Read the model definition and answer for the solid it produces. Units are mm, in the model's axes. A direction names the side the tool comes from. Coordinates: 2 decimals unless noted, no trailing zeros. Write each loop counter-clockwise with the first axis right and the second up, starting at its lowest first coordinate (ties: lowest second). Pieces come first, ordered by that corner, then holes.
from build123d import *

# Parameters (mm, degrees)
F1_DEPTH = 25.4


with BuildPart() as f1:
    # F0 (on Top) → F1 (new body)
    with BuildSketch(Plane.XY):
        Polygon((99.490069, 58.291368), (98.893963, 58.039229), (98.893963, 12.895242), (100.236297, 13.898268), (98.893963, 12.464104), (98.893963, -29.808243), (102.997907, -27.43528), (98.893963, -31.945548), (98.893963, -111.925168), (99.639752, -112.016652), (120.770343, 120.569244), (-22.619633, 111.361951), (105.815612, 95.447481), align=None)
        Polygon((98.893963, 12.895242), (98.893963, 58.039229), (-38.321942, 0), (97.543553, 35.373725), (5.177082, -57.132415), align=None)
        Polygon((100.236297, 13.898268), (98.893963, 12.895242), (98.893963, 12.464104), align=None)
        Polygon((98.893963, -29.808243), (98.893963, 12.464104), (12.658387, -79.670966), align=None)
        Polygon((102.997907, -27.43528), (98.893963, -29.808243), (98.893963, -31.945548), align=None)
        Polygon((98.893963, -111.925168), (98.893963, -31.945548), (33.426806, -103.894494), align=None)
        Polygon((99.639752, -112.016652), (98.893963, -111.925168), (98.893963, -120.225601), align=None)
    extrude(amount=F1_DEPTH)


solid = f1.part
Item 1: Find the intervals of material crossed by probe 1 along Y at (x, z) = (88, 15) (3 decimals); probe 2 along Y at (x, z) = (8.5, 14.25); probe 3 along Y at (x, z) = (92, 2), in increasing order.
Item 2: The part is cut by section B-B (y = -27). Give the vertices of the cut face in (x, z).
Item 3: Determine the mould class of faces 1 (the flat face through (82, 1, 25.4)), 2 (the flat face through (65.702, -107.854, 12.522)), 3 (the flat face through (52.01, -10.23, 12.52)) for opening direction Y: +Y half, -Y half, draft (parallel to the pull), parting line (faces both ways), or undercut.
Item 4: Given pin 1 (1.7 mm diameter, centred on y = -30.5, z = 8.5, fed in from -X); pin 2 (0.5 mm diameter, centred on y = 12.5, z = 17.5, fed in from -X); pin 3 (6 mm diameter, centred on x = 61, z = 20.5, fed in from +Y); pin 4 (6 mm diameter, centred on x = 68.5, y = -24, fed in from -Z), each flat-ended and moving along its own axis, determine where each tip first touches the part or whether it passes through.
Item 5: The part is cut by section A-A (x = -4). Give the vertices of the cut face in (y, z), and give its area (3 significant figures).
Item 6: The part is cut by section D-D (x = 82.5). Give the vertices of the cut face in (y, z), and give its area (3 significant figures).
Item 7: For faces 4 (the flat face through (82, 1, 0)), 5 (the flat face through (51.38, -22.61, 12.52)), 6 (the flat face through (98.894, -116, 13)), 7 (the flat face through (102.697, 77.13, 12.522)), determine the directions among +Z, -Z, +X, -X, +Y, -Y from which every point of the face is accessible in a straight line to the end or side of a thin tool.
Item 8: The part is cut by section C-C (x = 29.5). Give the vertices of the cut face in (y, z), and give its area (3 significant figures).
Answer:
1. probe 1: y = -110.589 to -43.918, -36.107 to 0.825, 4.755 to 25.816, 32.889 to 53.431, 97.655 to 118.465
1. probe 2: y = -54.65 to -53.8, 12.19 to 19.8, 107.51 to 113.36
1. probe 3: y = -111.08 to -39.52, -33.79 to 5.1, 7.74 to 29.82, 33.93 to 55.12, 97.16 to 118.72
2. outline: (35.26, 0) - (45.5, 0) - (45.5, 25.4) - (35.26, 25.4) - close; (61.96, 0) - (107.36, 0) - (107.36, 25.4) - (61.96, 25.4) - close
3. face 1: draft
3. face 2: -Y half
3. face 3: undercut
4. pin 1: stops at x = 30.92
4. pin 2: stops at x = -9.36
4. pin 3: stops at y = 116.92
4. pin 4: stops at z = 0
5. outline: (8.94, 0) - (14.52, 0) - (14.52, 25.4) - (8.94, 25.4) - close; (109.05, 0) - (112.56, 0) - (112.56, 25.4) - (109.05, 25.4) - close
5. area: 231 mm2
6. outline: (-109.91, 0) - (-49.96, 0) - (-49.96, 25.4) - (-109.91, 25.4) - close; (-39.29, 0) - (-5.05, 0) - (-5.05, 25.4) - (-39.29, 25.4) - close; (0.65, 0) - (20.31, 0) - (20.31, 25.4) - (0.65, 25.4) - close; (31.46, 0) - (51.1, 0) - (51.1, 25.4) - (31.46, 25.4) - close; (98.34, 0) - (118.11, 0) - (118.11, 25.4) - (98.34, 25.4) - close
6. area: 3,890 mm2
7. face 4: -Z, +X, -X, +Y, -Y
7. face 5: +Z, -Z
7. face 6: +Z, -Z, -X, -Y
7. face 7: +Z, -Z, -X
8. outline: (-69.93, 0) - (-61.68, 0) - (-61.68, 25.4) - (-69.93, 25.4) - close; (-38.96, 0) - (-32.77, 0) - (-32.77, 25.4) - (-38.96, 25.4) - close; (17.66, 0) - (28.69, 0) - (28.69, 25.4) - (17.66, 25.4) - close; (104.9, 0) - (114.71, 0) - (114.71, 25.4) - (104.9, 25.4) - close
8. area: 896 mm2
